Here's how the part is built. I have some questions about the finished solid (model axes, mm). Face numbers are marked on the shaded views. A direction names the side the tool comes from. Round coordinates to 2 decimals unless told otherwise and drop trailing zeros. Loops run counter-clockwise (first coordinate to the right, second up) from the corner with the lowest first, then second, coordinate; pieces in that order, holes last. Notation, with made-up numbers: (27.25, -30) -> (32.25, -30) arc R23 cw to (32.25, 8) -> close; hole circle Ø1 at (-26.75, 13.25). An arc over 180 degrees is marked (long way). One line per item, written item: value. Start each with the question number.
```python
from build123d import *

# Parameters (mm, degrees)
SKETCH1_R           = 4
BOSS_EXTRUDE1_DEPTH = 10
SKETCH2_W           = 50
SKETCH2_H           = 10
BOSS_EXTRUDE2_DEPTH = 15
SKETCH3_R           = 2.5
CUT_EXTRUDE1_DEPTH  = 11
SKETCH4_R           = 11
SKETCH4_R_2         = 4
BOSS_EXTRUDE3_DEPTH = 9


with BuildPart() as part:
    # Sketch1 → Boss-Extrude1 (new body)
    with BuildSketch(Plane.XY):
        with BuildLine():
            Line((25, 0), (25, 41.903210357))
            ThreePointArc((25, 41.903210357), (28.610974366, 58.852541508), (38.81677775, 72.858273892))
            ThreePointArc((38.81677775, 72.858273892), (42.138016249, 80.467397369), (38.567256581, 87.962666587))
            ThreePointArc((38.567256581, 87.962666587), (0, 102), (-38.567256581, 87.962666587))
            ThreePointArc((-38.567256581, 87.962666587), (-42.138016249, 80.467397369), (-38.81677775, 72.858273892))
            ThreePointArc((-38.81677775, 72.858273892), (-28.610974366, 58.852541508), (-25, 41.903210357))
            Line((-25, 41.903210357), (-25, 0))
            Line((-25, 0), (25, 0))
        make_face()
        with Locations((0, 42)):
            Circle(SKETCH1_R, mode=Mode.SUBTRACT)
        with BuildLine():
            ThreePointArc((28.925442436, 76.47199994), (0, 87), (-28.925442436, 76.47199994))
            ThreePointArc((-28.925442436, 76.47199994), (-35.9696027, 77.088284108), (-35.353318533, 84.132444372))
            ThreePointArc((-35.353318533, 84.132444372), (0, 97), (35.353318533, 84.132444372))
            ThreePointArc((35.353318533, 84.132444372), (35.9696027, 77.088284108), (28.925442436, 76.47199994))
        make_face(mode=Mode.SUBTRACT)
    extrude(amount=BOSS_EXTRUDE1_DEPTH)

    # Sketch2 → Boss-Extrude2 (add)
    with BuildSketch(Plane.XY.offset(10)):
        with Locations((0, 5)):
            Rectangle(SKETCH2_W, SKETCH2_H)
    extrude(amount=BOSS_EXTRUDE2_DEPTH)

    # Sketch3 → Cut-Extrude1 (cut, through all)
    with BuildSketch(Plane(origin=(0, 10, 0), x_dir=(1, 0, 0), z_dir=(0, 1, 0))):
        with Locations((-19, -17.5)):
            Circle(SKETCH3_R)
        with Locations((19, -17.5)):
            Circle(SKETCH3_R)
    extrude(amount=-CUT_EXTRUDE1_DEPTH, mode=Mode.SUBTRACT)

    # Sketch4 → Boss-Extrude3 (add)
    with BuildSketch(Plane.XY.offset(10)):
        with Locations((0, 42)):
            Circle(SKETCH4_R)
        with Locations((0, 42)):
            Circle(SKETCH4_R_2, mode=Mode.SUBTRACT)
    extrude(amount=BOSS_EXTRUDE3_DEPTH)


solid = part.part
```
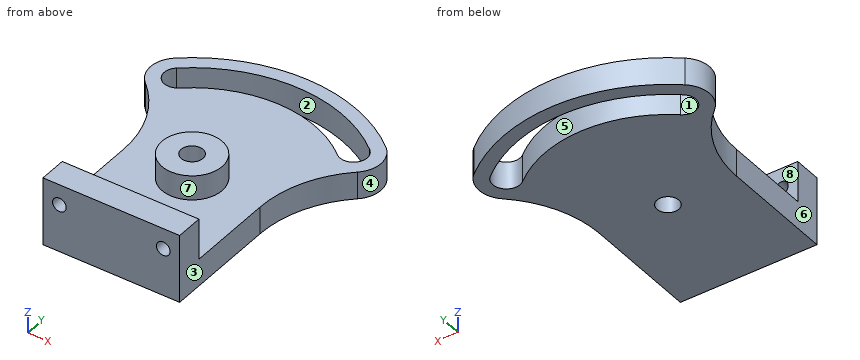
Q1. If I drill on line 1 along X through (y, z) = (7.25, 17.5); line 2 along Y through (x, z) = (0, 12.25); line 3 along Y through (x, z) = (0, 6), over which ranges is the centre line in solid material (lowest first)?
Q2. Which directions (+Z, -Z, +X, -X, +Y, -Y) give clear straight access to the entire face, cutting with the end or side of a thin tool? Please do the marked faces 5, 6, 7 and 8.
Q3. Will these pins go through, and if not, where does the flat tip stop? P1, Ø24, axis at x = -3, y = 38, coming from the +Z side; P2, Ø12, axis at y = 14.5, z = 6, coming from the +X side; P3, Ø12, axis at x = 6.5, z = 19, coming from the +Y side.
Q4. I want a section at A-A on z = 17.5. Please give me the cut outline in (x, y).
Q5. I want a section at C-C on x = 27. Please give me the cut outline in (y, z), plus the area to 3 significant figures.
Q6. I want a section at D-D on z = 7.25. Please give me the cut outline in (x, y).
Q7. I want a section at B-B on x = 0. Please give me the cut outline in (y, z).
Q8. If we mould it in two halves opening along Y, with no side actions, what happens to the marked faces 1, 2, 3 and 4? For each: released by +Y, released by -Y, zero draft, split by the parting line, or undercut.
Answers below:
1. line 1: x = -25 to -21.5, -16.5 to 16.5, 21.5 to 25
1. line 2: y = 0 to 10, 31 to 38, 46 to 53
1. line 3: y = 0 to 38, 46 to 87, 97 to 102
2. face 5: +Z, -Z
2. face 6: +Z, -Z, -X, -Y
2. face 7: +Z
2. face 8: +Z, +X, -X
3. P1: stops at z = 19
3. P2: stops at x = 25
3. P3: stops at y = 52.99
4. outline: (-25, 0) -> (-21.5, 0) -> (-21.5, 10) -> (-25, 10) -> close; (-16.5, 0) -> (16.5, 0) -> (16.5, 10) -> (-16.5, 10) -> close; circle Ø22 at (0, 42); (21.5, 0) -> (25, 0) -> (25, 10) -> (21.5, 10) -> close; hole circle Ø8 at (0, 42)
5. outline: (54.64, 0) -> (78, 0) -> (78, 10) -> (54.64, 10) -> close; (89.92, 0) -> (95.58, 0) -> (95.58, 10) -> (89.92, 10) -> close
5. area: 290 mm^2
6. outline: (-38.82, 72.86) arc R41.58 cw to (-25, 41.9) -> (-25, 0) -> (25, 0) -> (25, 41.9) arc R41.58 cw to (38.82, 72.86) arc R10 ccw to (38.57, 87.96) arc R60 ccw to (-38.57, 87.96) arc R10 ccw to start; hole (-35.35, 84.13) arc R5 ccw to (-28.93, 76.47) arc R45 cw to (28.93, 76.47) arc R5 ccw to (35.35, 84.13) arc R55 ccw to start; hole circle Ø8 at (0, 42)
7. outline: (0, 0) -> (38, 0) -> (38, 19) -> (31, 19) -> (31, 10) -> (10, 10) -> (10, 25) -> (0, 25) -> close; (46, 0) -> (87, 0) -> (87, 10) -> (53, 10) -> (53, 19) -> (46, 19) -> close; (97, 0) -> (102, 0) -> (102, 10) -> (97, 10) -> close
8. face 1: undercut
8. face 2: undercut
8. face 3: zero draft
8. face 4: split by the parting line
